```python
from build123d import *

# Parameters (mm, degrees)
F_01_HOUSING_PROFILE_W        = 240
F_01_HOUSING_PROFILE_H        = 180
F_01_HOUSING_PROFILE_R        = 7
F_01_HOUSING_BLOCK_DEPTH      = 120
F_02_FACE_BOSS_PROFILE_R      = 57.5
F_02_FACE_LOCATING_BOSS_DEPTH = 145


with BuildPart() as part:
    # 01_Housing_Profile → 01_Housing_Block (new body)
    with BuildSketch(Plane(origin=(0, 0, 0), x_dir=(1, 0, 0), z_dir=(0, 1, 0))):
        Rectangle(F_01_HOUSING_PROFILE_W, F_01_HOUSING_PROFILE_H)
        with Locations(Location((-85, -60, 0), (0, 0, 270))):
            Circle(F_01_HOUSING_PROFILE_R, mode=Mode.SUBTRACT)
        with Locations(Location((85, -60, 0), (0, 0, 270))):
            Circle(F_01_HOUSING_PROFILE_R, mode=Mode.SUBTRACT)
        with Locations(Location((-85, 60, 0), (0, 0, 270))):
            Circle(F_01_HOUSING_PROFILE_R, mode=Mode.SUBTRACT)
        with Locations(Location((85, 60, 0), (0, 0, 270))):
            Circle(F_01_HOUSING_PROFILE_R, mode=Mode.SUBTRACT)
    extrude(amount=F_01_HOUSING_BLOCK_DEPTH)

    # 02_Face_Boss_Profile → 02_Face_Locating_Boss (add)
    with BuildSketch(Plane(origin=(0, 0, 0), x_dir=(1, 0, 0), z_dir=(0, 1, 0))):
        with Locations(Location((0, 0, 0), (0, 0, 90))):
            Circle(F_02_FACE_BOSS_PROFILE_R)
    extrude(amount=F_02_FACE_LOCATING_BOSS_DEPTH)


solid = part.part
```
Geometry check sheet. Reference: the model listing, model coordinates, mm. A direction names the side the tool comes from. Round coordinates to 2 decimals unless told otherwise and drop trailing zeros. Loops run counter-clockwise (first coordinate to the right, second up) from the corner with the lowest first, then second, coordinate; pieces in that order, holes last. Notation, with made-up numbers: (59, -3) - (87, -3) arc R25 ccw to (87, 13) - close; hole circle Ø5 at (79, 57.5). An arc over 180 degrees is marked (long way). Write item = value, one per line. Start each with the question number.
1. Thickness scan on line 1 (X direction, y = 69, z = 60); line 2 (Z direction, x = -88, y = 81); line 3 (Y direction, x = -26, z = -54). Record the ranges inside material, lowest first.
2. Depth check by flat-ended pin: pin 1 (22.5 mm diameter, centred on x = 85, z = 60, fed in from +Y); pin 2 (4 mm diameter, centred on x = -5.5, y = 124, fed in from +Z). Enter the tip coordinate at first touch or a pass-through.
3. Set-up check for faces 4 (the face through (56.133, 132.325, 12.465)), 5 (the face through (91.94, 59.16, 59.09)): record each of +Z, -Z, +X, -X, +Y, -Y from which the full face is reachable in a straight line by a thin tool's end or side.
4. Section check C-C on x = -104. Enter the section's corners in (y, z).
5. Section check A-A on x = 0. Enter the section's corners in (y, z), then the cut area to 3 significant figures.
6. Mould release check, pull along X, two halves, no side actions. Record for faces 1 (the face through (-120, 59, 1)), 2 (the face through (-1, 145, 1)), 3 (the face through (91.94, 59.16, -60.91)): released by +X, released by -X, zero draft, split by the parting line, or undercut.
7. Section check B-B on z = 0. Enter the section's corners in (x, y).
Working result:
q1.line_1 = -120 to -92, -78 to 78, 92 to 120
q1.line_2 = -90 to -66.32, -53.68 to 53.68, 66.32 to 90
q1.line_3 = 0 to 120
q2.pin_1 = 120
q2.pin_2 = 57.39
q3.face_4 = +Y
q3.face_5 = +Y, -Y
q4.outline = (0, -90) - (120, -90) - (120, 90) - (0, 90) - close
q5.outline = (0, -90) - (120, -90) - (120, -57.5) - (145, -57.5) - (145, 57.5) - (120, 57.5) - (120, 90) - (0, 90) - close
q5.area = 24,500 mm^2
q6.face_1 = released by -X
q6.face_2 = zero draft
q6.face_3 = undercut
q7.outline = (-120, 0) - (120, 0) - (120, 120) - (57.5, 120) - (57.5, 145) - (-57.5, 145) - (-57.5, 120) - (-120, 120) - close
